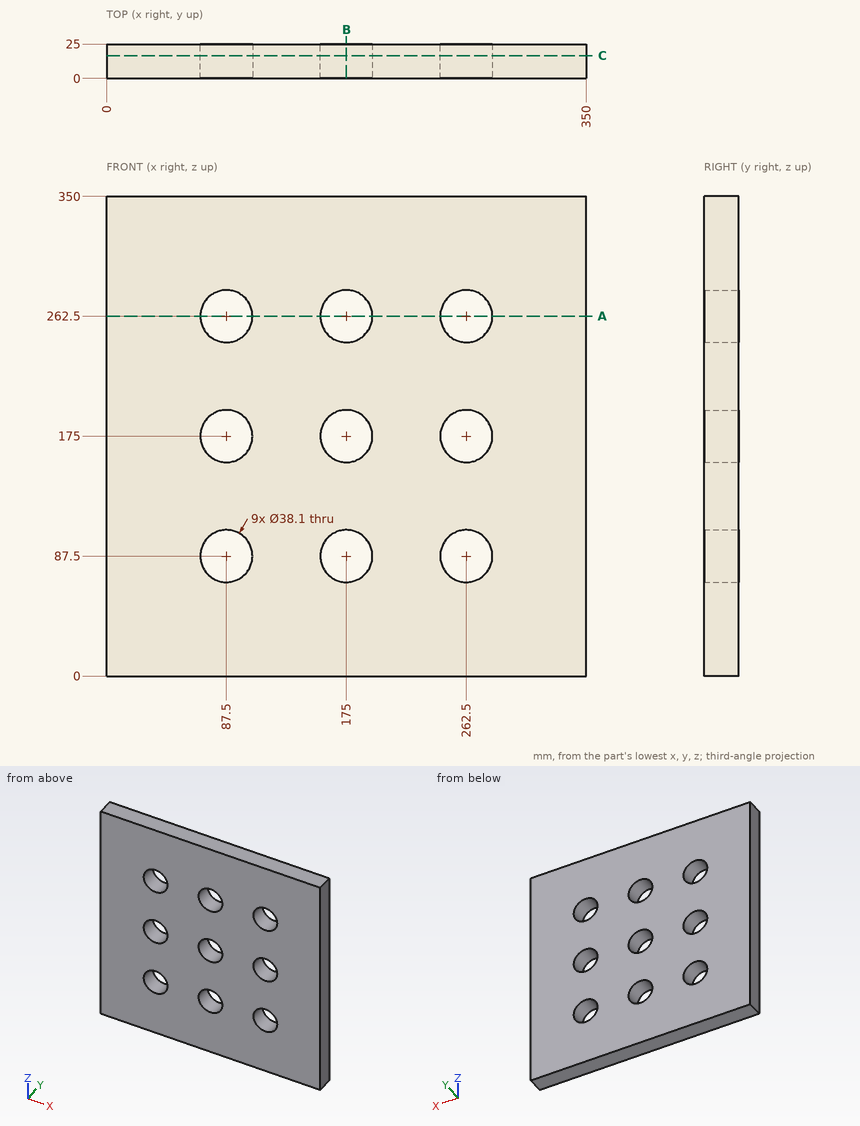
Drawing for the job (mm, zero at the part's lowest x, y, z). Give positions to 0.01 mm unless a question says otherwise; leave off trailing zeros. Loops run counter-clockwise (first coordinate to the right, second up) from the corner with the lowest first, then second, coordinate; pieces in that order, holes last.
1) Probe line 1 along Z through (x, y) = (175, 18.75); line 2 along X through (y, z) = (11, 275); line 3 along Z through (x, y) = (171.5, 10.5). List the from-to ranges inside material, lowest first.
Values follow:
line 1: z = 0 to 68.45, 106.55 to 155.95, 194.05 to 243.45, 281.55 to 350
line 2: x = 0 to 73.12, 101.88 to 160.62, 189.38 to 248.12, 276.88 to 350
line 3: z = 0 to 68.77, 106.23 to 156.27, 193.73 to 243.77, 281.23 to 350
2) Band-saw the part on C-C on y = 16.5. State how many separate pieces and enclosed holes the cut face has, then the cut area to 3 significant figures.
Values follow:
separate pieces: 1
enclosed holes: 9
area: 112,000 mm2
3) Band-saw the part on B-B on x = 175. List the corners of the cut face in (y, z).
Values follow:
outline: (0, 0) - (25, 0) - (25, 68.45) - (0, 68.45) - close; (0, 106.55) - (25, 106.55) - (25, 155.95) - (0, 155.95) - close; (0, 194.05) - (25, 194.05) - (25, 243.45) - (0, 243.45) - close; (0, 281.55) - (25, 281.55) - (25, 350) - (0, 350) - close
4) Band-saw the part on A-A on z = 262.5. List the corners of the cut face in (x, y), then the cut area to 3 significant figures.
Values follow:
outline: (0, 0) - (68.45, 0) - (68.45, 25) - (0, 25) - close; (106.55, 0) - (155.95, 0) - (155.95, 25) - (106.55, 25) - close; (194.05, 0) - (243.45, 0) - (243.45, 25) - (194.05, 25) - close; (281.55, 0) - (350, 0) - (350, 25) - (281.55, 25) - close
area: 5,890 mm2
